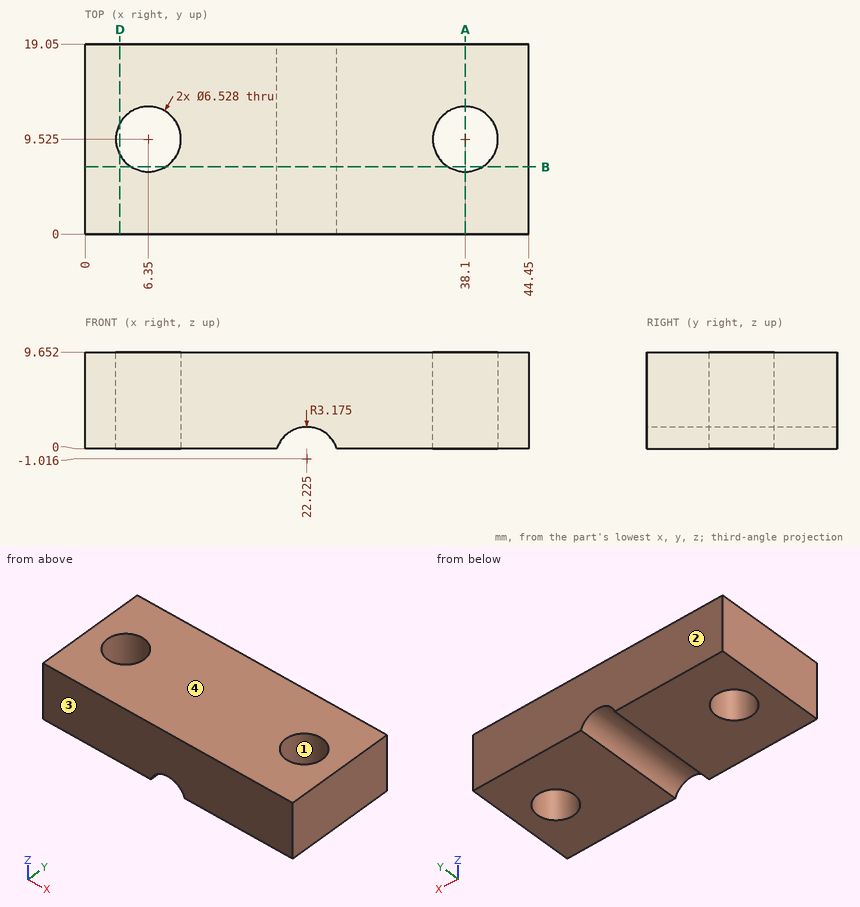
For this review, use the dimensioned drawing (mm, ordinates from the lowest corner) and the shaded views. Round coordinates to 2 decimals unless told otherwise and drop trailing zeros. Loops run counter-clockwise (first coordinate to the right, second up) from the corner with the lowest first, then second, coordinate; pieces in that order, holes last. Notation, with made-up numbers: (6, 3.25) -> (64, 3.25) arc R25 ccw to (64, 24.25) -> close; hole circle Ø8 at (-27.75, 77.25). An arc over 180 degrees is marked (long way). Write item = value, one per line. Start each with the question number.
Item 1: Take a section at A-A on x = 38.1. Give the boundary of the cut face in (y, z).
Item 2: To check wall thickness, follow L1, parallel to X at y = 9.5, z = 6.75; L2, parallel to Y at x = 6.35, z = 2.75; L3, parallel to X at y = 7.25, z = 8.25. State the ranges of each line that lie inside material, in increasing order.
Item 3: Take a section at D-D on x = 3.5. Give the boundary of the cut face in (y, z), plus the area to 3 significant figures.
Item 4: Take a section at B-B on y = 6.75. Count the separate pieces of the cut face and the enclosed holes in it, plus the area to 3 significant figures.
Item 5: Mouldability with a two-part tool opening along Y and no side actions: class the marked faces 1, 2, 3 and 4 as released by +Y, released by -Y, zero draft, split by the parting line, or undercut.
Item 6: Insertion check: pin 1 (2 mm diameter, centred on x = 22, y = 4.5, fed in from -Z). The pin has a flat end and moves straight along its axis. Give the tip position at first contact, or say it passes through.
Result:
q1.outline = (0, 0) -> (6.26, 0) -> (6.26, 9.65) -> (0, 9.65) -> close; (12.79, 0) -> (19.05, 0) -> (19.05, 9.65) -> (12.79, 9.65) -> close
q2.L1 = 0 to 3.09, 9.61 to 34.84, 41.36 to 44.45
q2.L2 = 0 to 6.26, 12.79 to 19.05
q2.L3 = 0 to 4.01, 8.69 to 35.76, 40.44 to 44.45
q3.outline = (0, 0) -> (7.93, 0) -> (7.93, 9.65) -> (0, 9.65) -> close; (11.12, 0) -> (19.05, 0) -> (19.05, 9.65) -> (11.12, 9.65) -> close
q3.area = 153 mm²
q4.separate_pieces = 3
q4.enclosed_holes = 0
q4.area = 353 mm²
q5.face_1 = undercut
q5.face_2 = released by +Y
q5.face_3 = released by -Y
q5.face_4 = zero draft
q6.pin_1 = 1.91
